from build123d import *

# Parameters (mm, degrees)
F1_DEPTH      = 17.5
F1_DEPTH_BACK = 17.5
F2_SIZE       = 15
F3_SIZE       = 7.5
F5_W          = 3
F5_H          = 92.5
F6_DEPTH      = 0.01
F7_W          = 3
F7_H          = 92.5
F8_DEPTH      = 0.01
F4_R          = 2.1
F9_DEPTH      = 3
F11_DEPTH     = 10
F13_DEPTH     = 10
F15_DEPTH     = 25


with BuildPart() as f1:
    # F0 (on Top) → F1 (new body, two sides)
    with BuildSketch(Plane.XY) as f1_sk:
        Polygon((147.5, -50), (147.5, 50), (-147.5, 50), (-147.5, -50), (-144.5, -50), (-144.5, -30), (144.5, -30), (144.5, -50), align=None)
    extrude(amount=F1_DEPTH)
    extrude(f1_sk.sketch, amount=-F1_DEPTH_BACK)

    # F2
    f2_edges = [f1.edges().sort_by_distance(p)[0] for p in [
        (0, -30, 17.5),
        (0, -30, -17.5),
    ]]
    chamfer(f2_edges, length=F2_SIZE)

    # F3
    f3_edges = [f1.edges().sort_by_distance(p)[0] for p in [
        (146, -50, 17.5),
        (146, -50, -17.5),
        (-146, -50, 17.5),
        (-146, -50, -17.5),
    ]]
    chamfer(f3_edges, length=F3_SIZE)

    # F5 (on face) → F6 (join)
    with BuildSketch(Plane.XY.offset(17.5)):
        with Locations((-146, 3.75)):
            Rectangle(F5_W, F5_H)
        with Locations((146, 3.75)):
            Rectangle(F5_W, F5_H)
    extrude(amount=F6_DEPTH)

    # F7 (on face) → F8 (join)
    with BuildSketch(Plane(origin=(0, 0, -17.5), x_dir=(1, 0, 0), z_dir=(0, 0, -1))):
        with Locations((-146, -3.75)):
            Rectangle(F7_W, F7_H)
        with Locations((146, -3.75)):
            Rectangle(F7_W, F7_H)
    extrude(amount=F8_DEPTH)

    # F4 (on face) → F9 (cut)
    with BuildSketch(Plane.YZ.offset(147.5)):
        with BuildLine():
            ThreePointArc((47.5, 0), (46.767767, 1.767767), (45, 2.5))
            Line((45, 2.5), (25, 2.5))
            ThreePointArc((25, 2.5), (23.232233, 1.767767), (22.5, 0))
            ThreePointArc((22.5, 0), (23.232233, -1.767767), (25, -2.5))
            Line((25, -2.5), (45, -2.5))
            ThreePointArc((45, -2.5), (46.767767, -1.767767), (47.5, 0))
        make_face()
        with Locations((35, 0)):
            Circle(F4_R, mode=Mode.SUBTRACT)
        with BuildLine():
            ThreePointArc((7.5, 0), (6.767767, 1.767767), (5, 2.5))
            Line((5, 2.5), (-15, 2.5))
            ThreePointArc((-15, 2.5), (-16.767767, 1.767767), (-17.5, 0))
            ThreePointArc((-17.5, 0), (-16.767767, -1.767767), (-15, -2.5))
            Line((-15, -2.5), (5, -2.5))
            ThreePointArc((5, -2.5), (6.767767, -1.767767), (7.5, 0))
        make_face()
        with Locations((-5, 0)):
            Circle(F4_R, mode=Mode.SUBTRACT)
    extrude(amount=-F9_DEPTH, mode=Mode.SUBTRACT)

    # F10 (on face) → F11 (cut)
    with BuildSketch(Plane.XY.offset(17.5)):
        with BuildLine():
            Line((141.5, 50), (-141.5, 50))
            Line((-141.5, 50), (-141.5, -2))
            ThreePointArc((-141.5, -2), (-138.571068, -9.071068), (-131.5, -12))
            Line((-131.5, -12), (131.5, -12))
            ThreePointArc((131.5, -12), (138.571068, -9.071068), (141.5, -2))
            Line((141.5, -2), (141.5, 50))
        make_face()
    extrude(amount=-F11_DEPTH, mode=Mode.SUBTRACT)

    # F12 (on face) → F13 (cut)
    with BuildSketch(Plane(origin=(0, 0, -17.5), x_dir=(1, 0, 0), z_dir=(0, 0, -1))):
        with BuildLine():
            Line((141.5, -50), (141.5, 2))
            ThreePointArc((141.5, 2), (138.571068, 9.071068), (131.5, 12))
            Line((131.5, 12), (-131.5, 12))
            ThreePointArc((-131.5, 12), (-138.571068, 9.071068), (-141.5, 2))
            Line((-141.5, 2), (-141.5, -50))
            Line((-141.5, -50), (141.5, -50))
        make_face()
    extrude(amount=-F13_DEPTH, mode=Mode.SUBTRACT)

    # F14 (on face) → F15 (cut)
    with BuildSketch(Plane.XY.offset(7.5)):
        with BuildLine():
            Line((121.5, 40), (-121.5, 40))
            ThreePointArc((-121.5, 40), (-128.571068, 37.071068), (-131.5, 30))
            Line((-131.5, 30), (-131.5, 8))
            ThreePointArc((-131.5, 8), (-128.571068, 0.928932), (-121.5, -2))
            Line((-121.5, -2), (121.5, -2))
            ThreePointArc((121.5, -2), (128.571068, 0.928932), (131.5, 8))
            Line((131.5, 8), (131.5, 30))
            ThreePointArc((131.5, 30), (128.571068, 37.071068), (121.5, 40))
        make_face()
    extrude(amount=-F15_DEPTH, mode=Mode.SUBTRACT)


solid = f1.part
Here's how the part is built. I have some questions about the finished solid (model axes, mm). A direction names the side the tool comes from. Round coordinates to 2 decimals unless told otherwise and drop trailing zeros. Loops run counter-clockwise (first coordinate to the right, second up) from the corner with the lowest first, then second, coordinate; pieces in that order, holes last. Notation, with made-up numbers: M -36.5,72 L -32.5,72 A14 cw -32.5,82 Z; hole C 74.5,31 d7. An arc over 180 degrees is marked long. Write each question's results on one line, items separated by ' | '. Start each with the question number.
(1) I want a section at C-C (y = -21). Please give me the cut outline in (x, z).
(2) If I drill on probe 1 along X at (y, z) = (29.5, 10); probe 2 along X at (y, z) = (9, -5); probe 3 along Z at (x, y) = (-46, -2.5), over which ranges is the centre line in solid material (lowest first)? Write a range as from..to.
(3) I want a section at A-A (x = -43). Please give me the cut outline in (y, z).
(4) Will these pins go through, and if not, where does the flat tip stop? P1, Ø8, axis at x = -32, y = -31.5, coming from the +Z side; P2, Ø4.5, axis at x = -4, z = 1, coming from the -Y side; P3, Ø10, axis at x = 39.5, y = 39.5, coming from the -Z side.
(5) On a 3-axis mill with a long thin cutter (end or side, diameter ignored), from which of +Z, -Z, +X, -X, +Y, -Y can I reach the whole of each face in a straight line? I mean faces 1 (the cylindrical face through (128.49, 0.85, 0.11)), 2 (the flat face through (-144.5, -37, 0)), 3 (the flat face through (-2, -30, 0)), 4 (the flat face through (144.5, -5.2, 2.3)), 5 (the flat face through (-1, 44, -7.5)). Say none if no direction works.
(6) Thinking about a two-plate mould opening in X: for faces 6 (the flat face through (147.5, -1, 4)), 7 (the flat face through (-146, -46, 14)), 8 (the flat face through (-131.5, 19, 0)), which applies, pulls with the +X half, pulls with the -X half, needs draft (parallel to the pull), parting line crosses it, or undercut?
Solved:
1) outline: M -147.5,-17.51 L -144.5,-17.51 L -144.5,-11.5 L 144.5,-11.5 L 144.5,-17.51 L 147.5,-17.51 L 147.5,17.51 L 144.5,17.51 L 144.5,11.5 L -144.5,11.5 L -144.5,17.51 L -147.5,17.51 Z
2) probe 1: x = -147.5..-141.5, 141.5..147.5 | probe 2: x = -147.5..-131.5, 131.5..147.5 | probe 3: z = -7.5..7.5
3) outline: M -30,-2.5 L -15,-17.5 L -12,-17.5 L -12,-7.5 L -2,-7.5 L -2,7.5 L -12,7.5 L -12,17.5 L -15,17.5 L -30,2.5 Z; M 40,-7.5 L 50,-7.5 L 50,7.5 L 40,7.5 Z
4) P1: stops at z = 5 | P2: stops at y = -30 | P3: stops at z = -7.5
5) face 1: +Z, -Z | face 2: -Y | face 3: +Z, -Z, -Y | face 4: +X | face 5: -Z, +Y
6) face 6: pulls with the +X half | face 7: needs draft | face 8: undercut
